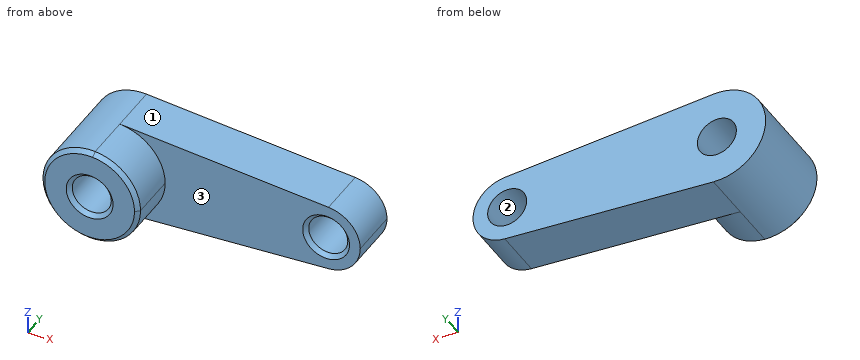
```python
from build123d import *

# Parameters (mm, degrees)
F0_R     = 10
F1_DEPTH = 25
F2_DEPTH = 50
F3_SIZE  = 2


with BuildPart() as f1:
    # F0 (on Front) → F1 (new body)
    with BuildSketch(Plane.XZ):
        with BuildLine():
            ThreePointArc((1.744186, 24.939082), (18.283936, 17.049858), (25, 0))
            ThreePointArc((25, 0), (18.283936, -17.049858), (1.744186, -24.939082))
            Line((1.744186, -24.939082), (108.72093, -17.457357))
            ThreePointArc((108.72093, -17.457357), (90, 0), (108.72093, 17.457357))
            Line((108.72093, 17.457357), (1.744186, 24.939082))
        make_face()
        with BuildLine():
            ThreePointArc((1.744186, -24.939082), (18.283936, -17.049858), (25, 0))
            ThreePointArc((25, 0), (18.283936, 17.049858), (1.744186, 24.939082))
            ThreePointArc((1.744186, 24.939082), (-25, 0), (1.744186, -24.939082))
        make_face()
        Circle(F0_R, mode=Mode.SUBTRACT)
        with BuildLine():
            ThreePointArc((125, 0), (120.298755, 11.934901), (108.72093, 17.457357))
            ThreePointArc((108.72093, 17.457357), (90, 0), (108.72093, -17.457357))
            ThreePointArc((108.72093, -17.457357), (120.298755, -11.934901), (125, 0))
        make_face()
        with Locations((107.5, 0)):
            Circle(F0_R, mode=Mode.SUBTRACT)
    extrude(amount=F1_DEPTH)

    # F0 (on Front) → F2 (join)
    with BuildSketch(Plane.XZ):
        with BuildLine():
            ThreePointArc((1.744186, -24.939082), (18.283936, -17.049858), (25, 0))
            ThreePointArc((25, 0), (18.283936, 17.049858), (1.744186, 24.939082))
            ThreePointArc((1.744186, 24.939082), (-25, 0), (1.744186, -24.939082))
        make_face()
        Circle(F0_R, mode=Mode.SUBTRACT)
    extrude(amount=F2_DEPTH)

    # F3
    f3_edges = [f1.edges().sort_by_distance(p)[0] for p in [
        (-10, -50, 0),
        (-1.744186, -50, 24.939082),
        (97.5, -25, 0),
    ]]
    chamfer(f3_edges, length=F3_SIZE)


solid = f1.part
```
For this review, take the finished solid that the model builds, in its own axes (mm). Face numbers are marked on the shaded views. Give positions to 0.01 mm unless a question says otherwise; leave off trailing zeros. Write each loop counter-clockwise with the first axis right and the second up, starting at its lowest first coordinate (ties: lowest second). Pieces come first, ordered by that corner, then holes.
Item 1: Take a section at A-A (y = -10.5). Give the boundary of the cut face in (x, z).
Item 2: Take a section at D-D (z = 4.5). Give the number of separate pieces and of enclosed holes in the cut face, and give its area (3 significant figures).
Item 3: The part is to be moulded in two halves that separate along X. For the marked faces 1, 2 and 3, say which applies: +X half, -X half, draft (parallel to the pull), parting line (faces both ways), or undercut.
Item 4: Wall thickness on probe 1 along Z at (x, y) = (0, -38); probe 2 along X at (y, z) = (-12, 1): over which ranges is each line inside the solid? List them lowest first.
Item 5: Insertion check: P1, Ø5, axis at y = -44, z = -8.5, coming from the +X side; P2, Ø6, axis at y = -36, z = 19, coming from the +X side; P3, Ø1.5, axis at x = 78, z = -2, coming from the -Y side. Each pin has a flat end and moves straight along its axis. Give the tip position at first contact, or say it passes through.
Item 6: Take a section at B-B (x = 0). Give the boundary of the cut face in (y, z), and give its area (3 significant figures).
Item 7: Take a section at C-C (y = -39.5). Give the boundary of the cut face in (x, z).
Established:
1. outline: (1.74, -24.94) - (108.72, -17.46) arc R17.5 ccw to (108.72, 17.46) - (1.74, 24.94) arc R25 ccw (long way) to start; hole circle Ø20 at (0, 0); hole circle Ø20 at (107.5, 0)
2. separate pieces: 3
2. enclosed holes: 0
2. area: 3,600 mm2
3. face 1: +X half
3. face 2: undercut
3. face 3: draft
4. probe 1: z = -25 to -10, 10 to 25
4. probe 2: x = -24.98 to -9.95, 9.95 to 97.55, 117.45 to 124.97
5. P1: stops at x = 24.27
5. P2: stops at x = 19.21
5. P3: stops at y = -25
6. outline: (-50, -23) - (-48, -25) - (0, -25) - (0, -10) - (-48, -10) - (-50, -12) - close; (-50, 12) - (-48, 10) - (0, 10) - (0, 25) - (-48, 25) - (-50, 23) - close
6. area: 1,490 mm2
7. outline: (1.74, -24.94) arc R25 ccw to (25, 0) arc R25 ccw to (1.74, 24.94) arc R25 ccw (long way) to start; hole circle Ø20 at (0, 0)
